Here's how the part is built. I have some questions about the finished solid (model axes, mm). A direction names the side the tool comes from. Give positions to 0.01 mm unless a question says otherwise; leave off trailing zeros. Loops run counter-clockwise (first coordinate to the right, second up) from the corner with the lowest first, then second, coordinate; pieces in that order, holes last. Notation, with made-up numbers: (34.5, 60.5) - (88.5, 60.5) arc R33 ccw to (88.5, 99.5) - close; hole circle Ø6 at (-4, 4.25). An arc over 180 degrees is marked (long way). Return JSON: item names as keys, results as strings. Group by question number.
(1) I need wall thicknesses on probe 1 along X at (y, z) = (1.15, 15.5); probe 2 along X at (y, z) = (-8, -12.5); probe 3 along Z at (x, y) = (-19, -13). Which ranges of each line are inside material? Lowest first, please. Write a range as [from, to].
(2) If we section it at A-A (y = -8): Please give me the cut outline in (x, z), then the cut area to 3 significant figures.
(3) On a 3-axis mill with a long thin cutter (end or side, diameter ignored), from which of +Z, -Z, +X, -X, +Y, -Y can I reach the whole of each face in a straight line? I mean faces 1 (the cylindrical face through (29.33, 1.23, -5.2)), 2 (the flat face through (-20.5, 1, 7)). Say none if no direction works.
(4) For P1, Ø2, axis at y = -19, z = 13.5, coming from the -X side; P2, Ø3, axis at y = 1, z = -1, coming from the +X side; P3, Ø8, axis at x = 25, z = 5.5, coming from the -Y side, each with a flat end and sliding along its axis, tell me the tip position at first contact or that it passes through.
(5) If we section it at C-C (x = 16): Please give me the cut outline in (y, z), then the cut area to 3 significant figures.
(6) If we mould it in two halves opening along Z, with no side actions, what happens to faces 3 (the flat face through (20.5, 1, 0)), 4 (the flat face through (20, -35, 18))? For each: released by +Z, released by -Z, zero draft, split by the parting line, or undercut.
(7) If we section it at B-B (z = 15.5): Please give me the cut outline in (x, y).
(8) If we section it at D-D (x = 25): Please give me the cut outline in (y, z).
```python
from build123d import *

# Parameters (mm, degrees)
SKETCH1_R                = 2.5
BOSS_EXTRUDE1_DEPTH      = 2.5
SKETCH4_R                = 3.5
SKETCH4_R_2              = 2
BOSS_EXTRUDE2_DEPTH      = 2.5
BOSS_EXTRUDE2_DEPTH_BACK = 35


with BuildPart() as part:
    # Sketch1 → Boss-Extrude1 (new body)
    with BuildSketch(Plane(origin=(0, 0, 0), x_dir=(1, 0, 0), z_dir=(0, 1, 0))):
        with BuildLine():
            Line((20.5, 10.5), (-20.5, 10.5))
            Line((-20.5, 10.5), (-20.5, 4))
            ThreePointArc((-20.5, 4), (-24.40287122, 1.76806345), (-28.520566145, 3.573204173))
            ThreePointArc((-28.520566145, 3.573204173), (-29.324072849, 5.171652721), (-29.350396575, 6.960498116))
            ThreePointArc((-29.350396575, 6.960498116), (-26.904940816, 10.941842627), (-22.5, 12.5))
            Line((-22.5, 12.5), (22.5, 12.5))
            ThreePointArc((22.5, 12.5), (26.904940816, 10.941842627), (29.350396575, 6.960498116))
            ThreePointArc((29.350396575, 6.960498116), (29.324072849, 5.171652721), (28.520566145, 3.573204173))
            ThreePointArc((28.520566145, 3.573204173), (25.737402548, 1.876578025), (22.5, 2.2557411))
            Line((22.5, 2.2557411), (22.5, -2.2557411))
            ThreePointArc((22.5, -2.2557411), (25.737402548, -1.876578025), (28.520566145, -3.573204173))
            ThreePointArc((28.520566145, -3.573204173), (29.324072849, -5.171652721), (29.350396575, -6.960498116))
            ThreePointArc((29.350396575, -6.960498116), (26.904940816, -10.941842627), (22.5, -12.5))
            Line((22.5, -12.5), (-22.5, -12.5))
            ThreePointArc((-22.5, -12.5), (-26.904940816, -10.941842627), (-29.350396575, -6.960498116))
            ThreePointArc((-29.350396575, -6.960498116), (-29.324072849, -5.171652721), (-28.520566145, -3.573204173))
            ThreePointArc((-28.520566145, -3.573204173), (-24.40287122, -1.76806345), (-20.5, -4))
            Line((-20.5, -4), (-20.5, -10.5))
            Line((-20.5, -10.5), (20.5, -10.5))
            Line((20.5, -10.5), (20.5, 10.5))
        make_face()
        with Locations((-25, 5.5)):
            Circle(SKETCH1_R, mode=Mode.SUBTRACT)
        with Locations((-25, -5.5)):
            Circle(SKETCH1_R, mode=Mode.SUBTRACT)
        with Locations((25, -5.5)):
            Circle(SKETCH1_R, mode=Mode.SUBTRACT)
        with Locations((25, 5.5)):
            Circle(SKETCH1_R, mode=Mode.SUBTRACT)
    extrude(amount=BOSS_EXTRUDE1_DEPTH)

    # Sketch4 → Boss-Extrude2 (add, two sides)
    with BuildSketch(Plane(origin=(0, 0, 0), x_dir=(1, 0, 0), z_dir=(0, 1, 0))) as boss_extrude2_sk:
        with Locations((-20.5, 15.5)):
            Circle(SKETCH4_R)
        with Locations((-20.5, 15.5)):
            Circle(SKETCH4_R_2, mode=Mode.SUBTRACT)
        with Locations((20.5, 15.5)):
            Circle(SKETCH4_R)
        with Locations((20.5, 15.5)):
            Circle(SKETCH4_R_2, mode=Mode.SUBTRACT)
        with Locations((-20.5, -15.5)):
            Circle(SKETCH4_R)
        with Locations((-20.5, -15.5)):
            Circle(SKETCH4_R_2, mode=Mode.SUBTRACT)
        with Locations((20.5, -15.5)):
            Circle(SKETCH4_R)
        with Locations((20.5, -15.5)):
            Circle(SKETCH4_R_2, mode=Mode.SUBTRACT)
    extrude(amount=BOSS_EXTRUDE2_DEPTH)
    extrude(boss_extrude2_sk.sketch, amount=-BOSS_EXTRUDE2_DEPTH_BACK)


solid = part.part
```
Values:
{
 "1": {"probe 1": "[-24, -22.5], [-18.5, -17], [17, 18.5], [22.5, 24]", "probe 2": "[-22.3, -18.7], [18.7, 22.3]", "probe 3": "[-18.66, -16.82], [-14.18, -12.34], [12.34, 14.18], [16.82, 18.66]"},
 "2": {"outline": "circle Ø7 at (-20.5, -15.5); circle Ø7 at (-20.5, 15.5); circle Ø7 at (20.5, -15.5); circle Ø7 at (20.5, 15.5); hole circle Ø4 at (-20.5, -15.5); hole circle Ø4 at (-20.5, 15.5); hole circle Ø4 at (20.5, -15.5); hole circle Ø4 at (20.5, 15.5)", "area": "104 mm2"},
 "3": {"face 1": "+X, +Y, -Y", "face 2": "+Y, -Y"},
 "4": {"P1": "x = -23.85", "P2": "x = 27.28", "P3": "y = 0"},
 "5": {"outline": "(0, -12.5) - (2.5, -12.5) - (2.5, -10.5) - (0, -10.5) - close; (0, 10.5) - (2.5, 10.5) - (2.5, 12.5) - (0, 12.5) - close", "area": "10.0 mm2"},
 "6": {"face 3": "undercut", "face 4": "zero draft"},
 "7": {"outline": "(-24, -35) - (-22.5, -35) - (-22.5, 2.5) - (-24, 2.5) - close; (-18.5, -35) - (-17, -35) - (-17, 2.5) - (-18.5, 2.5) - close; (17, -35) - (18.5, -35) - (18.5, 2.5) - (17, 2.5) - close; (22.5, -35) - (24, -35) - (24, 2.5) - (22.5, 2.5) - close"},
 "8": {"outline": "(0, -12.04) - (2.5, -12.04) - (2.5, -8) - (0, -8) - close; (0, -3) - (2.5, -3) - (2.5, -1.77) - (0, -1.77) - close; (0, 1.77) - (2.5, 1.77) - (2.5, 3) - (0, 3) - close; (0, 8) - (2.5, 8) - (2.5, 12.04) - (0, 12.04) - close"}
}
